Part model, mm, in its own coordinate system. A direction names the side the tool comes from. Round coordinates to 2 decimals unless told otherwise and drop trailing zeros. Write each loop counter-clockwise with the first axis right and the second up, starting at its lowest first coordinate (ties: lowest second). Pieces come first, ordered by that corner, then holes. Notation, with made-up numbers: M 88,74.25 L 106,74.25 A19 cw 106,100.25 Z; hole C -28,64.5 d3. An arc over 180 degrees is marked long. One line per question, with ' | ' between items. Start each with the question number.
1) Mould opens along X. For faces 6 (the face through (-21, 9.154, 12)), 7 (the face through (-20, -12.5, 0)), 8 (the face through (13.47, -13.4, -3.94)) say: pulls with the +X half, pulls with the -X half, needs draft (parallel to the pull), parting line crosses it, or undercut.
2) Tool access for faces 1 (the face through (-23, 2.509, 18)), 2 (the face through (0, 20, 0)), 3 (the face through (14, -14, -8)), 4 (the face through (20, 0, -8)), 5 (the face through (-22, -8, -1)): list every direction of +Z, -Z, +X, -X, +Y, -Y with a clear straight run to the whole face (end or side of a thin tool).
3) Saw through at C-C (x = 5.5). List the corners of the cut face in (y, z), plus the area to 3 significant figures.
4) Saw through at A-A (y = -16). List the corners of the cut face in (x, z).
5) Saw through at B-B (z = -9.25). List the corners of the cut face in (x, y).
6) Wall check: probe 1 along Z at (x, y) = (-20.2, -7); probe 2 along Z at (x, y) = (-20, 4); probe 3 along X at (y, z) = (-14, 9). Give the ranges that are in metal, low to high. Write a range as [from, to].
7) Saw through at D-D (y = -7). List the corners of the cut face in (x, z).
8) Drop flat-ended pins along their axis: pin 1 Ø12 at (y, z) = (-14, -21.5) entering from +X; pin 2 Ø4.5 at (x, z) = (-20.2, -24.25) entering from +Y; pin 3 Ø1 at (x, z) = (7, 8.5) entering from -Y; pin 4 Ø8 at (x, z) = (-20.12, -9.25) entering from -Y. Give the stop position or say it passes through.
```python
from build123d import *

# Parameters (mm, degrees)
F1_DEPTH       = 35
F3_D           = 5
F3_START       = 1.7550021
F3_START_2     = 1.8205079
F3_CBORE_D     = 10
F3_CBORE_DEPTH = 8
F4_W           = 22.4
F4_H           = 2
F5_DEPTH       = 12.5
F6_R           = 6
F7_DEPTH       = 8


with BuildPart() as f1:
    # F0 (on Top) → F1 (new body, symmetric)
    with BuildSketch(Plane.XY):
        with BuildLine():
            ThreePointArc((-17.3192642082, 2.5086026559), (17.5, 0), (-17.3192642082, -2.5086026559))
            Line((-17.3192642082, -2.5086026559), (-28.1192642082, -2.5086026559))
            Line((-28.1192642082, -2.5086026559), (-28.1192642082, -10.9086026559))
            ThreePointArc((-28.1192642082, -10.9086026559), (-25.7761184577, -16.5654569054), (-20.1192642082, -18.9086026559))
            Line((-20.1192642082, -18.9086026559), (-7.9192642082, -18.9086026559))
            ThreePointArc((-7.9192642082, -18.9086026559), (20.5, 0), (-7.9192642082, 18.9086026559))
            Line((-7.9192642082, 18.9086026559), (-20.1192642082, 18.9086026559))
            ThreePointArc((-20.1192642082, 18.9086026559), (-25.7761184577, 16.5654569054), (-28.1192642082, 10.9086026559))
            Line((-28.1192642082, 10.9086026559), (-28.1192642082, 2.5086026559))
            Line((-28.1192642082, 2.5086026559), (-17.3192642082, 2.5086026559))
        make_face()
    extrude(amount=F1_DEPTH, both=True)

    # F3 (through all)
    # its depths count from where the whole tool has entered the part; down to there all is cleared
    with Locations(Plane(origin=(0, 18.9086026559, 0), x_dir=(-1, 0, 0), z_dir=(0, 1, 0))):
        with Locations((20.1192642082, 24.25, -F3_START), (20.1192642082, 9.25, -F3_START), (20.1192642082, -9.25, -F3_START), (20.2, -24.2497827228, -F3_START_2)):
            CounterBoreHole(F3_D / 2, F3_CBORE_D / 2, F3_CBORE_DEPTH)

    # F4 (on Front) → F5 (cut, symmetric)
    with BuildSketch(Plane.XZ):
        with Locations((-16.9192642082, 0)):
            Rectangle(F4_W, F4_H)
    extrude(amount=F5_DEPTH, both=True, mode=Mode.SUBTRACT)

    # F6 (on Top) → F7 (cut)
    with BuildSketch(Plane.XY):
        with Locations((0, -25)):
            Circle(F6_R)
        with Locations((17.6776695297, -17.6776695297)):
            Circle(F6_R)
        with Locations((25, 0)):
            Circle(F6_R)
        with Locations((17.6776695297, 17.6776695297)):
            Circle(F6_R)
        with Locations((0, 25)):
            Circle(F6_R)
    extrude(amount=-F7_DEPTH, mode=Mode.SUBTRACT)


solid = f1.part
```
Answer key:
1) face 6: undercut | face 7: needs draft | face 8: pulls with the +X half
2) face 1: +Z, -Z, -X | face 2: +Y | face 3: +X, -Y | face 4: +X | face 5: -X
3) outline: M -19.75,-35 L -16.61,-35 L -16.61,35 L -19.75,35 Z; M 16.61,-35 L 19.75,-35 L 19.75,35 L 16.61,35 Z | area: 439 mm2
4) outline: M -26.29,-35 L -7.09,-35 L -7.09,35 L -26.29,35 Z; M 7.09,-35 L 12.82,-35 L 12.82,-8 L 11.92,-8 L 11.92,0 L 12.82,0 L 12.82,35 L 7.09,35 Z; hole C -20.2,-24.25 d5; hole C -20.12,-9.25 d5; hole C -20.12,9.25 d5; hole C -20.12,24.25 d5
5) outline: M -28.12,-10.91 A8 ccw -22.62,-18.51 L -22.62,-2.51 L -28.12,-2.51 Z; M -28.12,2.51 L -22.62,2.51 L -22.62,9.15 L -25.12,9.15 L -25.12,17.15 A8 ccw -28.12,10.91 Z; M -17.62,-18.91 L -7.92,-18.91 A20.5 ccw long -7.92,18.91 L -15.12,18.91 L -15.12,9.15 L -17.62,9.15 L -17.62,2.51 L -17.32,2.51 A17.5 cw long -17.32,-2.51 L -17.62,-2.51 Z
6) probe 1: z = [-35, -26.75], [-21.75, -11.75], [-6.75, -1], [1, 6.75], [11.75, 21.75], [26.75, 35] | probe 2: z = [-35, -26.74], [-21.76, -11.75], [-6.75, -1], [1, 6.75], [11.75, 21.75], [26.75, 35] | probe 3: x = [-27.5, -22.61], [-17.63, -10.5], [10.5, 14.97]
7) outline: M -28.12,-35 L -16.04,-35 L -16.04,-1 L -28.12,-1 Z; M -28.12,1 L -16.04,1 L -16.04,35 L -28.12,35 Z; M 16.04,-35 L 19.27,-35 L 19.27,35 L 16.04,35 Z; hole C -20.2,-24.25 d5; hole C -20.12,-9.25 d5; hole C -20.12,9.25 d5; hole C -20.12,24.25 d5
8) pin 1: stops at x = 18.87 | pin 2: passes through | pin 3: stops at y = -19.44 | pin 4: stops at y = -18.91
